Here's how the part is built. I have some questions about the finished solid (model axes, mm). A direction names the side the tool comes from. Give positions to 0.01 mm unless a question says otherwise; leave off trailing zeros. Loops run counter-clockwise (first coordinate to the right, second up) from the corner with the lowest first, then second, coordinate; pieces in that order, holes last. Notation, with made-up numbers: (75, -9) - (118, -9) arc R23 cw to (118, 21) - close; hole circle Ø3 at (16.5, -30.75). An arc over 180 degrees is marked (long way). Use a Markdown table: item, result.
from build123d import *

# Parameters (mm, degrees)
SKETCH2_R                 = 178
SKETCH2_R_2               = 100
BOSS_EXTRUDE1_DEPTH       = 3
SKETCH3_R                 = 178
SKETCH3_R_2               = 175
BOSS_EXTRUDE2_DEPTH       = 60
CUT_EXTRUDE2_START        = -25
CUT_EXTRUDE2_DEPTH        = 25
BOSS_EXTRUDE4_START       = -50
BOSS_EXTRUDE4_DEPTH       = 50
BOSS_EXTRUDE5_START       = 3
BOSS_EXTRUDE5_DEPTH       = 3
BOSS_EXTRUDE15_REACH      = 346.25
BOSS_EXTRUDE15_END_RADIUS = 175
BOSS_EXTRUDE16_REACH      = 263.713
SKETCH15_W                = 3.001191186
SKETCH15_H                = 49
FILLET2_START             = 104.957134107
FILLET2_DEPTH             = 3.001191186
SKETCH16_R                = 178
CUT_EXTRUDE3_DEPTH        = 73
CUT_EXTRUDE4_REACH        = 200.073
SKETCH17_R                = 2.25


with BuildPart() as part:
    # Sketch2 → Boss-Extrude1 (new body)
    with BuildSketch(Plane(origin=(0, 0, 0), x_dir=(1, 0, 0), z_dir=(0, 1, 0))):
        with Locations(Location((0, 0, 0), (0, 0, 270))):
            Circle(SKETCH2_R)
        with Locations(Location((0, 0, 0), (0, 0, 270))):
            Circle(SKETCH2_R_2, mode=Mode.SUBTRACT)
    extrude(amount=BOSS_EXTRUDE1_DEPTH)

    # Sketch3 → Boss-Extrude2 (add)
    with BuildSketch(Plane(origin=(0, 3, 0), x_dir=(1, 0, 0), z_dir=(0, 1, 0))):
        with Locations(Location((0, 0, 0), (0, 0, 270))):
            Circle(SKETCH3_R)
        with Locations(Location((0, 0, 0), (0, 0, 270))):
            Circle(SKETCH3_R_2, mode=Mode.SUBTRACT)
    extrude(amount=BOSS_EXTRUDE2_DEPTH)

    # Sketch5 → Cut-Extrude2 (cut)
    with BuildSketch(Plane(origin=(0, 3, 0), x_dir=(1, 0, 0), z_dir=(0, 1, 0)).offset(CUT_EXTRUDE2_START)):
        with BuildLine():
            Line((174.470835958, 13.59880142), (99.697620548, 7.770743669))
            ThreePointArc((99.697620548, 7.770743669), (99.924376542, 3.888312311), (100, 0))
            ThreePointArc((100, 0), (97.525905257, -22.106510438), (90.226043925, -43.11914885))
            Line((90.226043925, -43.11914885), (157.895576869, -75.458510488))
            ThreePointArc((157.895576869, -75.458510488), (170.6703342, -38.686393266), (175, 0))
            ThreePointArc((175, 0), (174.867658949, 6.804546543), (174.470835958, 13.59880142))
        make_face()
    extrude(amount=CUT_EXTRUDE2_DEPTH, mode=Mode.SUBTRACT)

    # Sketch16 → Cut-Extrude3 (cut)
    with BuildSketch(Plane(origin=(0, -10, 0), x_dir=(1, 0, 0), z_dir=(0, 1, 0))):
        Circle(SKETCH16_R)
    extrude(amount=CUT_EXTRUDE3_DEPTH, mode=Mode.SUBTRACT)


with BuildPart() as body_2:
    # Sketch8 → Boss-Extrude4 (new body)
    with BuildSketch(Plane(origin=(0, -10, 0), x_dir=(1, 0, 0), z_dir=(0, 1, 0)).offset(BOSS_EXTRUDE4_START)):
        with BuildLine():
            Line((157.895576869, -75.458510488), (97.444127439, -46.568680758))
            ThreePointArc((97.444127439, -46.568680758), (98.081576263, -45.210666859), (98.700100465, -43.843929662))
            ThreePointArc((98.700100465, -43.843929662), (106.176660799, -19.761495426), (107.86500381, 5.398236111))
            ThreePointArc((107.86500381, 5.398236111), (107.779614919, 6.895984919), (107.673430191, 8.392403162))
            ThreePointArc((107.673430191, 8.392403162), (107.546470116, 9.88720211), (107.39875919, 11.380093344))
            Line((107.39875919, 11.380093344), (104.40664299, 11.14687847))
            ThreePointArc((104.40664299, 11.14687847), (103.227309111, -19.212564998), (93.405095457, -47.963404203))
            Line((93.405095457, -47.963404203), (156.578799716, -78.15420321))
            ThreePointArc((156.578799716, -78.15420321), (157.242965096, -76.80917867), (157.895576869, -75.458510488))
        make_face()
    extrude(amount=BOSS_EXTRUDE4_DEPTH)

    # Sketch9 → Boss-Extrude5 (add)
    with BuildSketch(Plane(origin=(0, -10, 0), x_dir=(-1, 0, 0), z_dir=(0, -1, 0)).offset(BOSS_EXTRUDE5_START)):
        with BuildLine():
            ThreePointArc((-93.405095457, -47.963404203), (-103.227309111, -19.212564998), (-104.40664299, 11.14687847))
            Line((-104.40664299, 11.14687847), (-174.212075233, 16.587731699))
            ThreePointArc((-174.212075233, 16.587731699), (-172.045515184, -32.020941663), (-156.578799716, -78.15420321))
            Line((-156.578799716, -78.15420321), (-93.405095457, -47.963404203))
        make_face()
    extrude(amount=-BOSS_EXTRUDE5_DEPTH)


with BuildPart() as body_3:
    # Boss-Extrude15: up to this cylinder (the profile starts inside it)
    boss_extrude15_end = Plane(origin=(0, -35.052685, 0), z_dir=(0, -1, 0)) * Cylinder(BOSS_EXTRUDE15_END_RADIUS, 1043.5, mode=Mode.PRIVATE)
    # Sketch14 → Boss-Extrude15 (new, up to the surface)
    with BuildSketch(Plane(origin=(104.6397653, 0, -8.155949853), x_dir=(0, 1, 0), z_dir=(0.9969762054751131, 0, -0.07770743668687732)), mode=Mode.PRIVATE) as boss_extrude15_sk1:
        with BuildLine():
            Line((-56, -33.149626863), (-59, -33.149626863))
            add(Edge.make_bspline(
                [(-13, -3), (-13, -3.252742632), (-13.017835017, -3.772139773), (-13.118535688, -4.696081698), (-13.354753506, -5.728289796), (-13.790711815, -6.796346653), (-14.57235228, -8.073596542), (-15.969031451, -9.501150583), (-18.417965946, -11.02187183), (-21.560218655, -12.309547439), (-26.464579206, -13.73861764), (-33.523749843, -15.121678766), (-42.302010507, -16.833830818), (-49.062318848, -19.008877457), (-53.702980916, -21.83051429), (-56.611293913, -24.732512094), (-58.237380526, -27.905736518), (-58.80960896, -30.443459169), (-58.972930909, -31.962804263), (-59, -32.756631085), (-59, -33.149626863)],
                knots=[0, 0, 0, 0, 0.015625, 0.03125, 0.0625, 0.09375, 0.125, 0.1875, 0.25, 0.3125, 0.375, 0.5, 0.625, 0.75, 0.8125, 0.875, 0.9375, 0.96875, 0.984375, 1, 1, 1, 1], degree=3))
            Line((-13, -3), (-10, -3))
            add(Edge.make_bspline(
                [(-10, -3), (-10, -24.167074489), (-56, -11.982552374), (-56, -33.149626863)],
                knots=[0, 0, 0, 0, 1, 1, 1, 1], degree=3))
        make_face()
    boss_extrude15_tool1 = extrude(boss_extrude15_sk1.sketch, amount=BOSS_EXTRUDE15_REACH, mode=Mode.PRIVATE) & boss_extrude15_end
    add(boss_extrude15_tool1.solids().sort_by_distance((103.281222, -35.052685, -25.585884))[0])

    # Sketch15 → Boss-Extrude16 (add, up to next)
    with BuildSketch(Plane(origin=(-0.23312231, 0, -2.990928616), x_dir=(-0.9969762054751131, 0, 0.07770743668687734), z_dir=(-0.07770743668687734, 0, -0.9969762054751131)), mode=Mode.PRIVATE) as boss_extrude16_sk1:
        with Locations((-106.4577297, -34.5)):
            Rectangle(SKETCH15_W, SKETCH15_H)
    boss_extrude16_tool1 = extrude(boss_extrude16_sk1.sketch, amount=BOSS_EXTRUDE16_REACH, mode=Mode.PRIVATE) - body_3.part

    add(body_2.part)  # Boss-Extrude16 merges body 2
    add(boss_extrude16_tool1.solids().sort_by_distance((105.902701, -34.5, -11.263486))[0])

    # Fillet2: read off the stored shape, not the designer's step
    # Fillet2 outline → Fillet2 (add)
    with BuildSketch(Plane(origin=(0, 0, 0), x_dir=(0, 1, 0), z_dir=(0.9969762054751131, 0, -0.07770743668687731)).offset(FILLET2_START)):
        with BuildLine():
            Line((-59, -3), (-60, -3))
            ThreePointArc((-60, -3), (-59.253205655, -5.122830966), (-59, -7.358898944))
            Line((-59, -7.358898944), (-59, -3))
        make_face()
    extrude(amount=FILLET2_DEPTH)

    # Sketch17 → Cut-Extrude4 (cut, up to next)
    with BuildSketch(Plane(origin=(0, -10, 0), x_dir=(1, 0, 0), z_dir=(0, 1, 0)), mode=Mode.PRIVATE) as cut_extrude4_sk1:
        with Locations(Location((133.270755038, -21.538473754, 0), (0, 0, 270))):
            Circle(SKETCH17_R)
    cut_extrude4_tool1 = extrude(cut_extrude4_sk1.sketch, amount=-CUT_EXTRUDE4_REACH, mode=Mode.PRIVATE) & body_3.part
    add(cut_extrude4_tool1.solids().sort_by_distance((133.270755, -10, 21.538474))[0], mode=Mode.SUBTRACT)


solid = body_3.part
(1) If I drill on line 1 (Y direction, x = 145.5, z = 5); line 2 (Z direction, x = 154, y = -48.5); line 3 (X direction, y = -50, z = 0), over which ranges is the centre line in solid material (lowest first)?
A:
| item | result |
|---|---|
| line 1 | -13 to -10 |
| line 2 | -34.4 to -31.1, 73.6 to 76.92 |
| line 3 | 105 to 108 |
(2) Will these pins go through, and if not, where does the flat tip stop? pin 1 (2 mm diameter, centred on x = 128.5, y = -45.5, fed in from +Z); pin 2 (10 mm diameter, centred on x = 139.5, y = -18, fed in from -Z); pin 3 (8 mm diameter, centred on x = 128, z = -13.5, fed in from -Y).
A:
| item | result |
|---|---|
| pin 1 | z = 65.21 |
| pin 2 | z = -26.81 |
| pin 3 | y = -14.24 |
(3) Suppose I cut it at A-A on z = 18. Write out the boundary of the cut face in (x, y), plus the area to 3 significant figures.
A:
| item | result |
|---|---|
| outline | (103.45, -60) - (106.49, -60) - (106.49, -13) - (174.07, -13) - (174.07, -10) - (103.45, -10) - close |
| area | 355 mm2 |
(4) On a 3-axis mill with a long thin cutter (end or side, diameter ignored), from which of +Z, -Z, +X, -X, +Y, -Y can I reach the whole of each face in a straight line? I mean faces 5 (the face through (105, -59, -28)), 6 (the face through (103.77, -40.91, -19.29)), 7 (the face through (134.933, -57.479, -43.767)), 8 (the face through (137, -13, 19)). Say none if no direction works.
A:
| item | result |
|---|---|
| face 5 | -Z, +X, -X, -Y |
| face 6 | -X, +Y, -Y |
| face 7 | -Z, -X, +Y, -Y |
| face 8 | +X, -Y |
(5) We'd pull the mould along Z, two halves only. Please class faces 1 (the face through (131.074, -11.479, 21.051)), 2 (the face through (143, -10, 20)), 3 (the face through (124.55, -35.35, 62.847)), 4 (the face through (105.72, -59.26, -13.35)): pulls with the +Z half, pulls with the -Z half, needs draft (parallel to the pull), parting line crosses it, or undercut.
A:
| item | result |
|---|---|
| face 1 | undercut |
| face 2 | needs draft |
| face 3 | pulls with the +Z half |
| face 4 | pulls with the -Z half |
